The listing builds one solid part. Answer for the finished solid, in the listing's coordinates (mm). A direction names the side the tool comes from. Coordinates: 2 decimals unless noted, no trailing zeros. Loops run counter-clockwise (first coordinate to the right, second up) from the corner with the lowest first, then second, coordinate; pieces in that order, holes last. Notation, with made-up numbers: M -10,16 L 10,16 A10 cw 10,35 Z; hole C 71,5.5 d2. An arc over 180 degrees is marked long. Return JSON: item names as keys, results as strings. Group by question number.
1. Section A-A (x = -36.5) is taken. Write down the section's boundary in (y, z).
2. Straight lines are drawn through the part: L1, parallel to Z at x = -27.5, y = 7; L2, parallel to X at y = 25, z = 2.5; L3, parallel to X at y = -14, z = 4.5. For each, find the intervals that lie inside material, in ascending order. Write a range as from..to.
3. Section C-C (z = 19) is taken. Write down the section's boundary in (x, y).
4. Which of the six approach directions +Z, -Z, +X, -X, +Y, -Y give full straight-line access (tool end or side, diameter ignored) to faces 1 (the face through (-22, 11, 0)), 2 (the face through (10.89, 18.73, 8.65)), 3 (the face through (-34.57, -2.858, 11.972))?
5. Given P1, Ø2.5, axis at x = -41.5, z = 5, coming from the -Y side; P2, Ø8, axis at x = -34, z = 9.5, coming from the -Y side; P3, Ø6, axis at y = 22, z = 18.5, coming from the -X side, each flat-ended and moving along its own axis, determine where each tip first touches the part or whether it passes through.
6. Section B-B (y = 23.5) is taken. Write down the section's boundary in (x, z).
7. Section D-D (y = 9.5) is taken. Write down the section's boundary in (x, z).
```python
from build123d import *

# Parameters (mm, degrees)
BOSS_EXTRUDE1_DEPTH      = 10
FILLET1_R                = 10
FILLET2_R                = 5
BOSS_EXTRUDE2_DEPTH      = 10
BOSS_EXTRUDE2_DEPTH_BACK = 40
SKETCH2_R                = 7
BOSS_EXTRUDE3_START      = -5
SKETCH3_R                = 5
BOSS_EXTRUDE3_DEPTH      = 15
CHAMFER1_SIZE            = 2.5
BOSS_EXTRUDE4_DEPTH      = 18
BOSS_EXTRUDE4_DEPTH_BACK = 10
SKETCH4_R                = 13
SKETCH5_R                = 14
BOSS_EXTRUDE5_DEPTH      = 4


with BuildPart() as part:
    # Sketch1 → Boss-Extrude1 (new body)
    with BuildSketch(Plane.XY):
        Polygon((-58.818184361, 21.563458262), (11.382033939, 21.563458262), (11.382033939, 7.563458262), (-34.282866194, -6.436541738), (-58.818184361, -6.436541738), align=None)
    extrude(amount=BOSS_EXTRUDE1_DEPTH)

    # Fillet1
    fillet1_edges = [part.edges().sort_by_distance(p)[0] for p in [
        (-58.818184361, 21.563458262, 5),
        (-58.818184361, -6.436541738, 5),
    ]]
    fillet(fillet1_edges, radius=FILLET1_R)

    # Fillet2
    fillet2_edges = [part.edges().sort_by_distance(p)[0] for p in [
        (11.382033939, 21.563458262, 5),
        (11.382033939, 7.563458262, 5),
        (-34.282866194, -6.436541738, 5),
    ]]
    fillet(fillet2_edges, radius=FILLET2_R)

    # Sketch2 → Boss-Extrude2 (add, two sides: drawn at the far end of the back side and taken through both)
    with BuildSketch(Plane(origin=(0, 21.563458262, 0), x_dir=(1, 0, 0), z_dir=(0, 1, 0)).offset(-BOSS_EXTRUDE2_DEPTH_BACK)):
        with Locations(Location((-48.818184361, -5, 0), (0, 0, 270))):
            Circle(SKETCH2_R)
    extrude(amount=BOSS_EXTRUDE2_DEPTH + BOSS_EXTRUDE2_DEPTH_BACK)

    # Sketch3 → Boss-Extrude3 (add)
    with BuildSketch(Plane(origin=(0, 21.563458262, 0), x_dir=(1, 0, 0), z_dir=(0, 1, 0)).offset(BOSS_EXTRUDE3_START)):
        with Locations(Location((6.382033939, -5, 0), (0, 0, 270))):
            Circle(SKETCH3_R)
    extrude(amount=BOSS_EXTRUDE3_DEPTH)

    # Chamfer1
    chamfer1_edges = [part.edges().sort_by_distance(p)[0] for p in [
        (-48.818184361, -18.436541738, -2),
        (-48.818184361, 31.563458262, -2),
        (6.382033939, 31.563458262, 0),
    ]]
    chamfer(chamfer1_edges, length=CHAMFER1_SIZE)

    # Sketch4 → Boss-Extrude4 (add, two sides: drawn at the far end of the back side and taken through both)
    with BuildSketch(Plane.XY.offset(10).offset(-BOSS_EXTRUDE4_DEPTH_BACK)):
        with Locations((-43.919204876, 7.563458262)):
            Circle(SKETCH4_R)
    extrude(amount=BOSS_EXTRUDE4_DEPTH + BOSS_EXTRUDE4_DEPTH_BACK)

    # Sketch5 → Boss-Extrude5 (add)
    with BuildSketch(Plane.XY.offset(10)):
        with Locations(Location((-43.919204876, 7.563458262, 0), (0, 0, 134.415308597))):
            Circle(SKETCH5_R)
    extrude(amount=BOSS_EXTRUDE5_DEPTH)


solid = part.part
```
Worked out:
{
 "1": {"outline": "M -6.44,0 L 21.56,0 L 21.56,10 L 19.44,10 L 19.44,14 L 18.24,14 L 18.24,28 L -3.11,28 L -3.11,14 L -4.31,14 L -4.31,10 L -6.44,10 Z"},
 "2": {"L1": "0..10", "L2": "-55.36..-42.28, 2.05..10.71", "L3": "-55.8..-41.84"},
 "3": {"outline": "C -43.92,7.56 d26"},
 "4": {"face 1": "-Z, +X, +Y, -Y", "face 2": "+Z, +X, +Y", "face 3": "+Z"},
 "5": {"P1": "y = -16.87", "P2": "y = -6.44", "P3": "x = -50.1"},
 "6": {"outline": "C -48.82,5 d14; C 6.38,5 d10"},
 "7": {"outline": "M -58.82,0 L -53.72,0 A7 ccw -43.92,0 L 11.06,0 L 11.06,10 L -30.05,10 L -30.05,14 L -31.06,14 L -31.06,28 L -56.77,28 L -56.77,14 L -57.78,14 L -57.78,10 L -58.82,10 Z"}
}
